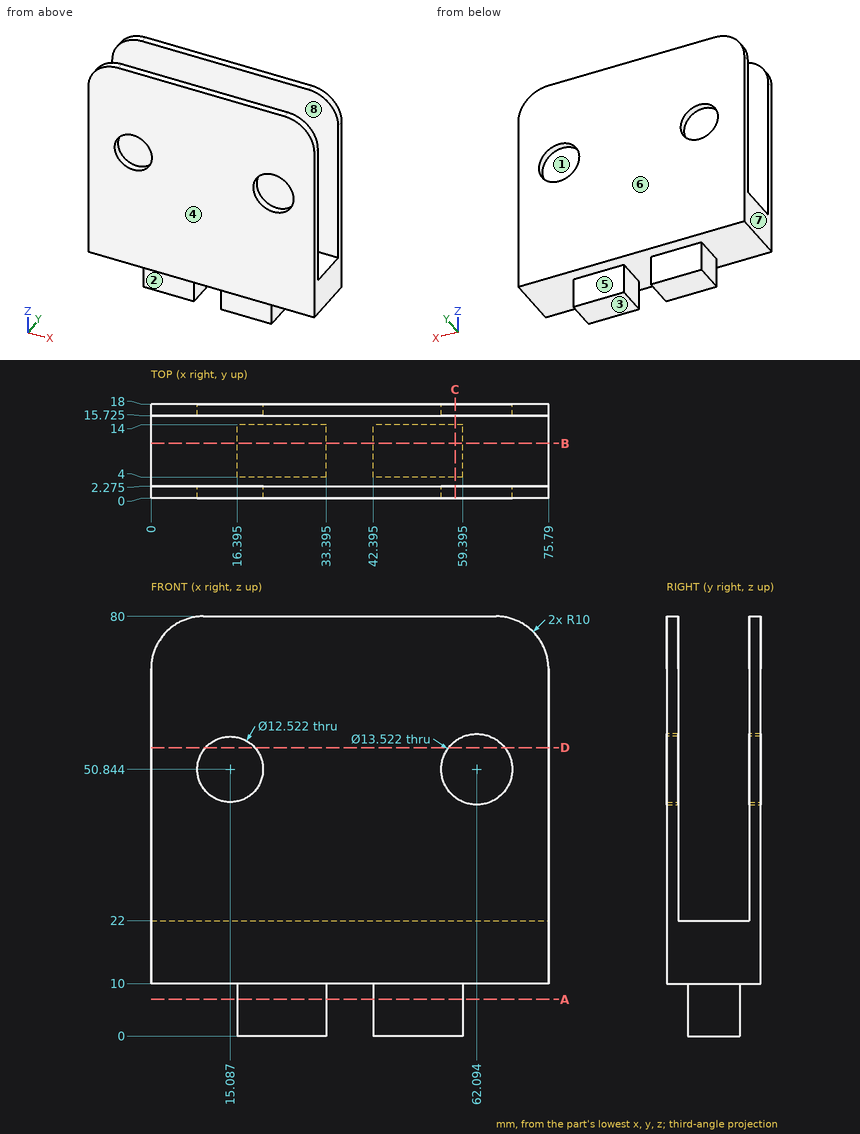
Design review of the part shown in the three views and the two pictorial views. Dimensions are in mm from the part's minimum x, y and z. A direction names the side the tool comes from. Round coordinates to 2 decimals unless told otherwise and drop trailing zeros. Write each loop counter-clockwise with the first axis right and the second up, starting at its lowest first coordinate (ties: lowest second). Pieces come first, ordered by that corner, then holes. Notation, with made-up numbers: (2, 47.25) -> (35, 47.25) arc R24 cw to (35, 80.25) -> close; hole circle Ø1 at (40, 74). An arc over 180 degrees is marked (long way). One line per question, with ' | ' between items. Start each with the question number.
1) Add section C-C (x = 58). Write out the cut boundary in (y, z) (1 decimal).
2) Add section A-A (z = 7). Write out the cut boundary in (x, y) (1 decimal), and give its area (3 significant figures).
3) Wall thickness on line 1 along Y through (x, z) = (35, 71) (1 decimal); line 2 along Z through (x, y) = (15, 2); line 3 along Z through (x, y) = (47.5, 1.5): over which ranges is each line inside the solid? List them lowest first.
4) Machinability: for the marked faces 1, 2, 3, 4 and 5, which of the approach directions +Z, -Z, +X, -X, +Y, -Y give a long, thin tool a straight path to every point of the face, cutting with its end or side? Answer none if there is none.
5) For pin 1 Ø8 at (x, y) = (16.5, 10.5) entering from +Z; pin 2 Ø5 at (x, z) = (49.5, 7) entering from +Y; pin 3 Ø5 at (x, z) = (52, 5.5) entering from -Y, all flat-tipped, find the tip position at first contact; note any pin that passes through.
6) Mouldability with a two-part tool opening along Y and no side actions: class the marked faces 6, 7 and 8 as +Y half, -Y half, draft (parallel to the pull), parting line (faces both ways), or undercut.
7) Add section B-B (y = 10.5). Write out the cut boundary in (x, z) (1 decimal).
8) Add section D-D (z = 55). Write out the cut boundary in (x, y) (1 decimal), and give its area (3 significant figures).
Reported:
1) outline: (0, 10) -> (4, 10) -> (4, 0) -> (14, 0) -> (14, 10) -> (18, 10) -> (18, 45.5) -> (15.7, 45.5) -> (15.7, 22) -> (2.3, 22) -> (2.3, 45.5) -> (0, 45.5) -> close; (0, 56.2) -> (2.3, 56.2) -> (2.3, 80) -> (0, 80) -> close; (15.7, 56.2) -> (18, 56.2) -> (18, 80) -> (15.7, 80) -> close
2) outline: (16.4, 4) -> (33.4, 4) -> (33.4, 14) -> (16.4, 14) -> close; (42.4, 4) -> (59.4, 4) -> (59.4, 14) -> (42.4, 14) -> close | area: 340 mm²
3) line 1: y = 0 to 2.3, 15.7 to 18 | line 2: z = 10 to 44.58, 57.1 to 80 | line 3: z = 10 to 80
4) face 1: +Z, +X, -X | face 2: -Z, +X, -X, -Y | face 3: -Z, +X, -X, +Y, -Y | face 4: +Z, -Z, +X, -X, -Y | face 5: -Z, +X, -X, +Y
5) pin 1: stops at z = 22 | pin 2: stops at y = 14 | pin 3: stops at y = 4
6) face 6: +Y half | face 7: draft | face 8: undercut
7) outline: (0, 10) -> (16.4, 10) -> (16.4, 0) -> (33.4, 0) -> (33.4, 10) -> (42.4, 10) -> (42.4, 0) -> (59.4, 0) -> (59.4, 10) -> (75.8, 10) -> (75.8, 22) -> (0, 22) -> close
8) outline: (0, 0) -> (10.4, 0) -> (10.4, 2.3) -> (0, 2.3) -> close; (0, 15.7) -> (10.4, 15.7) -> (10.4, 18) -> (0, 18) -> close; (19.8, 0) -> (56.8, 0) -> (56.8, 2.3) -> (19.8, 2.3) -> close; (19.8, 15.7) -> (56.8, 15.7) -> (56.8, 18) -> (19.8, 18) -> close; (67.4, 0) -> (75.8, 0) -> (75.8, 2.3) -> (67.4, 2.3) -> close; (67.4, 15.7) -> (75.8, 15.7) -> (75.8, 18) -> (67.4, 18) -> close | area: 254 mm²
